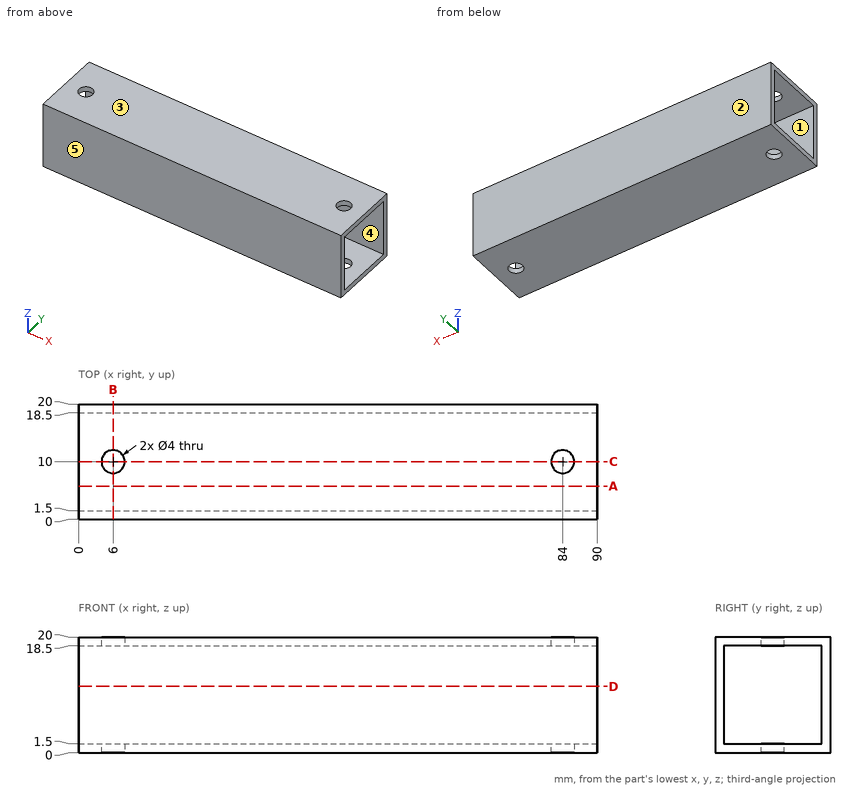
The drawing under review shows one solid part. Ordinate dimensions are in mm from its lowest x, y, z. A direction names the side the tool comes from. Round coordinates to 2 decimals unless told otherwise and drop trailing zeros. Loops run counter-clockwise (first coordinate to the right, second up) from the corner with the lowest first, then second, coordinate; pieces in that order, holes last. Notation, with made-up numbers: (54.25, 3.5) - (82.25, 3.5) arc R31 ccw to (82.25, 37.5) - close; hole circle Ø10 at (20.25, 21). An arc over 180 degrees is marked (long way). Use a Markdown table: item, result. Add a question column.
Q1. Add section C-C (y = 10). State the section outline as (x, z) points.
Q2. Add section B-B (x = 6). State the section outline as (y, z) points.
Q3. Machinability: for the marked faces 1 and 2, which of the approach directions +Z, -Z, +X, -X, +Y, -Y give a long, thin tool a straight path to every point of the face, cutting with its end or side? Answer none if there is none.
Q4. Add section A-A (y = 5.75). State the section outline as (x, z) points.
Q5. Insertion check: pin 1 Ø2.5 at (x, y) = (84, 10) entering from +Z. The pin has a flat end and moves straight along its axis. Give the tip position at first contact, or say it passes through.
Q6. For probe 1 along Y at (x, z) = (6, 0.35); probe 2 along Y at (x, z) = (85, 18), list the stretches that pass through material, from the lowest coordinate up.
Q7. The part is to be moulded in two halves that separate along Z. For the marked faces 3, 4 and 5, say which applies: pulls with the +Z half, pulls with the -Z half, needs draft (parallel to the pull), parting line crosses it, or undercut.
Worked answers:
| question | item | result |
|---|---|---|
| 1 | outline | (0, 0) - (4, 0) - (4, 1.5) - (0, 1.5) - close; (0, 18.5) - (4, 18.5) - (4, 20) - (0, 20) - close; (8, 0) - (82, 0) - (82, 1.5) - (8, 1.5) - close; (8, 18.5) - (82, 18.5) - (82, 20) - (8, 20) - close; (86, 0) - (90, 0) - (90, 1.5) - (86, 1.5) - close; (86, 18.5) - (90, 18.5) - (90, 20) - (86, 20) - close |
| 2 | outline | (0, 0) - (8, 0) - (8, 1.5) - (1.5, 1.5) - (1.5, 18.5) - (8, 18.5) - (8, 20) - (0, 20) - close; (12, 0) - (20, 0) - (20, 20) - (12, 20) - (12, 18.5) - (18.5, 18.5) - (18.5, 1.5) - (12, 1.5) - close |
| 3 | face 1 | +X, -X |
| 3 | face 2 | +Z, -Z, +X, -X, +Y |
| 4 | outline | (0, 0) - (90, 0) - (90, 1.5) - (0, 1.5) - close; (0, 18.5) - (90, 18.5) - (90, 20) - (0, 20) - close |
| 5 | pin 1 | through |
| 6 | probe 1 | 0 to 8, 12 to 20 |
| 6 | probe 2 | 0 to 1.5, 18.5 to 20 |
| 7 | face 3 | pulls with the +Z half |
| 7 | face 4 | undercut |
| 7 | face 5 | needs draft |
